```python
from build123d import *

# Parameters (mm, degrees)
SKETCH2_W                            = 83
SKETCH2_H                            = 30
BOSS_EXTRUDE1_DEPTH                  = 120
CUT_EXTRUDE1_DEPTH                   = 28
CUT_EXTRUDE4_REACH                   = 122
SKETCH10_R                           = 3
SKETCH10_R_2                         = 1.6
BOSS_EXTRUDE2_DEPTH                  = 5
SKETCH13_R                           = 5
BOSS_EXTRUDE_CC3D_SUPPORT_DEPTH      = 2
SKETCH10_3_R                         = 1.6
CUT_EXTRUDE_CC3D_ROUND_DEPTH         = 10
CUT_EXTRUDE_CC3D_ROUND_DEPTH_BACK    = 5
SKETCH14_R                           = 1.6
CUT_EXTRUDE_BOTTOM_HEX_CORNERS_DEPTH = 3.5
SKETCH14_5_R                         = 1.6
CUT_EXTRUDE_BOTTOM_HEX_CC3D_DEPTH    = 2.5
SKETCH14_4_R                         = 1.6
CUT_EXTRUDE_BOTTOM_ROUND_DEPTH       = 31
CUT_EXTRUDE12_DEPTH                  = 25
CUT_HOLES_RIGHT_REACH                = 85
SKETCH8_R                            = 4
CUT_HOLES_LEFT_START                 = -83
SKETCH8_4_R                          = 4
CUT_HOLES_LEFT_DEPTH                 = 2
FILLET1_4MM_R                        = 4
CUT_EXTRUDE14_REACH                  = 122
SKETCH15_R                           = 3
CUT_EXTRUDE15_START                  = -120
SKETCH15_2_R                         = 3
CUT_EXTRUDE15_DEPTH                  = 2


with BuildPart() as part:
    # Sketch2 → Boss-Extrude1 (new body)
    with BuildSketch(Plane.XY):
        Rectangle(SKETCH2_W, SKETCH2_H)
    extrude(amount=-BOSS_EXTRUDE1_DEPTH)

    # Sketch4 → Cut-Extrude1 (cut)
    with BuildSketch(Plane(origin=(0, 15, 0), x_dir=(1, 0, 0), z_dir=(0, 1, 0))):
        with BuildLine():
            Line((-24.5, 118), (-31, 118))
            ThreePointArc((-31, 118), (-33.48959236, 111.98959236), (-39.5, 109.5))
            Line((-39.5, 109.5), (-39.5, 10.5))
            ThreePointArc((-39.5, 10.5), (-33.48959236, 8.01040764), (-31, 2))
            Line((-31, 2), (-24.5, 2))
            Line((-24.5, 2), (-24.5, 55))
            Line((-24.5, 55), (-22.5, 55))
            Line((-22.5, 55), (-22.5, 2))
            Line((-22.5, 2), (22.5, 2))
            Line((22.5, 2), (22.5, 55))
            Line((22.5, 55), (24.5, 55))
            Line((24.5, 55), (24.5, 2))
            Line((24.5, 2), (31, 2))
            ThreePointArc((31, 2), (33.48959236, 8.01040764), (39.5, 10.5))
            Line((39.5, 10.5), (39.5, 109.5))
            ThreePointArc((39.5, 109.5), (33.48959236, 111.98959236), (31, 118))
            Line((31, 118), (24.5, 118))
            Line((24.5, 118), (24.5, 65))
            Line((24.5, 65), (22.5, 65))
            Line((22.5, 65), (22.5, 118))
            Line((22.5, 118), (-22.5, 118))
            Line((-22.5, 118), (-22.5, 65))
            Line((-22.5, 65), (-24.5, 65))
            Line((-24.5, 65), (-24.5, 118))
        make_face()
    extrude(amount=-CUT_EXTRUDE1_DEPTH, mode=Mode.SUBTRACT)

    # Sketch6 → Cut-Extrude4 (cut, up to next)
    with BuildSketch(Plane.XY, mode=Mode.PRIVATE) as cut_extrude4_sk1:
        with BuildLine():
            Line((-2, 2), (2, 2))
            ThreePointArc((2, 2), (4, 0), (2, -2))
            Line((2, -2), (-2, -2))
            ThreePointArc((-2, -2), (-4, 0), (-2, 2))
        make_face()
    cut_extrude4_tool1 = extrude(cut_extrude4_sk1.sketch, amount=-CUT_EXTRUDE4_REACH, mode=Mode.PRIVATE) & part.part
    add(cut_extrude4_tool1.solids().sort_by_distance((0, 0, 0))[0], mode=Mode.SUBTRACT)

    # Sketch10 → Boss-Extrude2 (add)
    with BuildSketch(Plane(origin=(0, -13, 0), x_dir=(1, 0, 0), z_dir=(0, 1, 0))):
        with Locations((-15.25, 100.25)):
            Circle(SKETCH10_R)
        with Locations((-15.25, 100.25)):
            Circle(SKETCH10_R_2, mode=Mode.SUBTRACT)
        with Locations((15.25, 100.25)):
            Circle(SKETCH10_R)
        with Locations((15.25, 100.25)):
            Circle(SKETCH10_R_2, mode=Mode.SUBTRACT)
        with Locations((15.25, 69.75)):
            Circle(SKETCH10_R)
        with Locations((15.25, 69.75)):
            Circle(SKETCH10_R_2, mode=Mode.SUBTRACT)
        with Locations((-15.25, 69.75)):
            Circle(SKETCH10_R)
        with Locations((-15.25, 69.75)):
            Circle(SKETCH10_R_2, mode=Mode.SUBTRACT)
    extrude(amount=BOSS_EXTRUDE2_DEPTH)

    # Sketch13 → Boss-Extrude-cc3d-support (add)
    with BuildSketch(Plane(origin=(0, -13, 0), x_dir=(1, 0, 0), z_dir=(0, 1, 0))):
        with Locations((-15.25, 100.25)):
            Circle(SKETCH13_R)
        with Locations((15.25, 100.25)):
            Circle(SKETCH13_R)
        with Locations((-15.25, 69.75)):
            Circle(SKETCH13_R)
        with Locations((15.25, 69.75)):
            Circle(SKETCH13_R)
    extrude(amount=BOSS_EXTRUDE_CC3D_SUPPORT_DEPTH)

    # Sketch10_3 → Cut-Extrude-cc3d-round (cut, two sides)
    with BuildSketch(Plane(origin=(0, -13, 0), x_dir=(1, 0, 0), z_dir=(0, 1, 0))) as cut_extrude_cc3d_round_sk:
        with Locations((-15.25, 100.25)):
            Circle(SKETCH10_3_R)
        with Locations((15.25, 100.25)):
            Circle(SKETCH10_3_R)
        with Locations((-15.25, 69.75)):
            Circle(SKETCH10_3_R)
        with Locations((15.25, 69.75)):
            Circle(SKETCH10_3_R)
    extrude(amount=CUT_EXTRUDE_CC3D_ROUND_DEPTH, mode=Mode.SUBTRACT)
    extrude(cut_extrude_cc3d_round_sk.sketch, amount=-CUT_EXTRUDE_CC3D_ROUND_DEPTH_BACK, mode=Mode.SUBTRACT)

    # Sketch14 → Cut-Extrude-bottom-hex-corners (cut)
    with BuildSketch(Plane.XZ.offset(15)):
        Polygon((-39.5, -113.063655198), (-39.5, -116.354551733), (-36.65, -118), (-33.8, -116.354551733), (-33.8, -113.063655198), (-36.65, -111.418206931), align=None)
        with Locations((-36.65, -114.709103466)):
            Circle(SKETCH14_R, mode=Mode.SUBTRACT)
        Polygon((33.8, -113.063655198), (33.8, -116.354551733), (36.65, -118), (39.5, -116.354551733), (39.5, -113.063655198), (36.65, -111.418206931), align=None)
        with Locations((36.65, -114.709103466)):
            Circle(SKETCH14_R, mode=Mode.SUBTRACT)
        Polygon((33.8, -3.645448267), (33.8, -6.936344802), (36.65, -8.581793069), (39.5, -6.936344802), (39.5, -3.645448267), (36.65, -2), align=None)
        with Locations((36.65, -5.290896534)):
            Circle(SKETCH14_R, mode=Mode.SUBTRACT)
        Polygon((-39.5, -3.645448267), (-39.5, -6.936344802), (-36.65, -8.581793069), (-33.8, -6.936344802), (-33.8, -3.645448267), (-36.65, -2), align=None)
        with Locations((-36.65, -5.290896534)):
            Circle(SKETCH14_R, mode=Mode.SUBTRACT)
    extrude(amount=-CUT_EXTRUDE_BOTTOM_HEX_CORNERS_DEPTH, mode=Mode.SUBTRACT)

    # Sketch14_5 → Cut-Extrude-bottom-hex-cc3d (cut)
    with BuildSketch(Plane.XZ.offset(15)):
        Polygon((-18.1, -98.604551733), (-18.1, -101.895448267), (-15.25, -103.540896534), (-12.4, -101.895448267), (-12.4, -98.604551733), (-15.25, -96.959103466), align=None)
        with Locations((-15.25, -100.25)):
            Circle(SKETCH14_5_R, mode=Mode.SUBTRACT)
        Polygon((-18.1, -68.104551733), (-18.1, -71.395448267), (-15.25, -73.040896534), (-12.4, -71.395448267), (-12.4, -68.104551733), (-15.25, -66.459103466), align=None)
        with Locations((-15.25, -69.75)):
            Circle(SKETCH14_5_R, mode=Mode.SUBTRACT)
        Polygon((12.4, -68.104551733), (12.4, -71.395448267), (15.25, -73.040896534), (18.1, -71.395448267), (18.1, -68.104551733), (15.25, -66.459103466), align=None)
        with Locations((15.25, -69.75)):
            Circle(SKETCH14_5_R, mode=Mode.SUBTRACT)
        Polygon((12.4, -98.604551733), (12.4, -101.895448267), (15.25, -103.540896534), (18.1, -101.895448267), (18.1, -98.604551733), (15.25, -96.959103466), align=None)
        with Locations((15.25, -100.25)):
            Circle(SKETCH14_5_R, mode=Mode.SUBTRACT)
    extrude(amount=-CUT_EXTRUDE_BOTTOM_HEX_CC3D_DEPTH, mode=Mode.SUBTRACT)

    # Sketch14_4 → Cut-Extrude-bottom-round (cut, through all)
    with BuildSketch(Plane.XZ.offset(15)):
        with Locations((-36.65, -5.290896534)):
            Circle(SKETCH14_4_R)
        with Locations((36.65, -5.290896534)):
            Circle(SKETCH14_4_R)
        with Locations((36.65, -114.709103466)):
            Circle(SKETCH14_4_R)
        with Locations((-36.65, -114.709103466)):
            Circle(SKETCH14_4_R)
    extrude(amount=-CUT_EXTRUDE_BOTTOM_ROUND_DEPTH, mode=Mode.SUBTRACT)

    # Sketch4_5 → Cut-Extrude12 (cut)
    with BuildSketch(Plane(origin=(0, 15, 0), x_dir=(1, 0, 0), z_dir=(0, 1, 0))):
        with BuildLine():
            Line((-31, 118), (-39.5, 118))
            Line((-39.5, 118), (-39.5, 109.5))
            ThreePointArc((-39.5, 109.5), (-33.48959236, 111.98959236), (-31, 118))
        make_face()
        with BuildLine():
            Line((39.5, 118), (31, 118))
            ThreePointArc((31, 118), (33.48959236, 111.98959236), (39.5, 109.5))
            Line((39.5, 109.5), (39.5, 118))
        make_face()
        with BuildLine():
            Line((39.5, 2), (39.5, 10.5))
            ThreePointArc((39.5, 10.5), (33.48959236, 8.01040764), (31, 2))
            Line((31, 2), (39.5, 2))
        make_face()
        with BuildLine():
            ThreePointArc((-31, 2), (-33.48959236, 8.01040764), (-39.5, 10.5))
            Line((-39.5, 10.5), (-39.5, 2))
            Line((-39.5, 2), (-31, 2))
        make_face()
    extrude(amount=-CUT_EXTRUDE12_DEPTH, mode=Mode.SUBTRACT)

    # Sketch8 → Cut-Holes-Right (cut, up to next)
    with BuildSketch(Plane(origin=(41.5, 0, 0), x_dir=(0, 0, -1), z_dir=(1, 0, 0)), mode=Mode.PRIVATE) as cut_holes_right_sk1:
        with Locations((30, 0)):
            Circle(SKETCH8_R)
    cut_holes_right_tool1 = extrude(cut_holes_right_sk1.sketch, amount=-CUT_HOLES_RIGHT_REACH, mode=Mode.PRIVATE) & part.part
    add(cut_holes_right_tool1.solids().sort_by_distance((41.5, 0, -30))[0], mode=Mode.SUBTRACT)
    # Sketch8 → Cut-Holes-Right (cut, up to next)
    with BuildSketch(Plane(origin=(41.5, 0, 0), x_dir=(0, 0, -1), z_dir=(1, 0, 0)), mode=Mode.PRIVATE) as cut_holes_right_sk2:
        with Locations((90, 0)):
            Circle(SKETCH8_R)
    cut_holes_right_tool2 = extrude(cut_holes_right_sk2.sketch, amount=-CUT_HOLES_RIGHT_REACH, mode=Mode.PRIVATE) & part.part
    add(cut_holes_right_tool2.solids().sort_by_distance((41.5, 0, -90))[0], mode=Mode.SUBTRACT)

    # Sketch8_4 → Cut-Holes-Left (cut)
    with BuildSketch(Plane(origin=(41.5, 0, 0), x_dir=(0, 0, -1), z_dir=(1, 0, 0)).offset(CUT_HOLES_LEFT_START)):
        with Locations((30, 0)):
            Circle(SKETCH8_4_R)
        with Locations((90, 0)):
            Circle(SKETCH8_4_R)
    extrude(amount=CUT_HOLES_LEFT_DEPTH, mode=Mode.SUBTRACT)

    # Fillet1_4mm
    fillet1_4mm_edges = [part.edges().sort_by_distance(p)[0] for p in [
        (41.5, 0, -120),
        (-39.5, 2.5, -118),
        (39.5, 2.5, -118),
        (39.5, 2.5, -2),
        (-41.5, 0, -120),
        (-39.5, 2.5, -2),
        (41.5, 0, 0),
        (-41.5, 0, 0),
    ]]
    fillet(fillet1_4mm_edges, radius=FILLET1_4MM_R)

    # Sketch15 → Cut-Extrude14 (cut, up to next)
    with BuildSketch(Plane.XY, mode=Mode.PRIVATE) as cut_extrude14_sk1:
        with Locations((-32.5, 0)):
            Circle(SKETCH15_R)
    cut_extrude14_tool1 = extrude(cut_extrude14_sk1.sketch, amount=-CUT_EXTRUDE14_REACH, mode=Mode.PRIVATE) & part.part
    add(cut_extrude14_tool1.solids().sort_by_distance((-32.5, 0, 0))[0], mode=Mode.SUBTRACT)
    # Sketch15 → Cut-Extrude14 (cut, up to next)
    with BuildSketch(Plane.XY, mode=Mode.PRIVATE) as cut_extrude14_sk2:
        with Locations((32.5, 0)):
            Circle(SKETCH15_R)
    cut_extrude14_tool2 = extrude(cut_extrude14_sk2.sketch, amount=-CUT_EXTRUDE14_REACH, mode=Mode.PRIVATE) & part.part
    add(cut_extrude14_tool2.solids().sort_by_distance((32.5, 0, 0))[0], mode=Mode.SUBTRACT)

    # Sketch15_2 → Cut-Extrude15 (cut)
    with BuildSketch(Plane.XY.offset(CUT_EXTRUDE15_START)):
        with Locations((-32.5, 0)):
            Circle(SKETCH15_2_R)
        with Locations((32.5, 0)):
            Circle(SKETCH15_2_R)
    extrude(amount=CUT_EXTRUDE15_DEPTH, mode=Mode.SUBTRACT)


solid = part.part
```
Build history of the part. All positions in model axes, mm. A direction names the side the tool comes from. Round coordinates to 2 decimals unless told otherwise and drop trailing zeros. Loops run counter-clockwise (first coordinate to the right, second up) from the corner with the lowest first, then second, coordinate; pieces in that order, holes last.
Item 1: Saw through at A-A (z = -30). List the corners of the cut face in (x, y), then the cut area to 3 significant figures.
Item 2: Which spindle directions (+Z, -Z, +X, -X, +Y, -Y) get a long thin tool onto all of the face, cutting with end or side? Do faces 1 (the face through (-41, 0, -86)), 2 (the face through (16.69, -13.77, -67.29)), 3 (the face through (-29, 1, -118)). Say none if no direction does.
Item 3: Pin check, flat tips, straight feed: P1, Ø2.5, axis at x = -36.65, z = -5.29, coming from the +Y side; P2, Ø8, axis at x = 0, z = -27, coming from the +Y side; P3, Ø3, axis at x = 15, z = -102.5, coming from the +Y side; P4, Ø4, axis at x = -15.25, z = -69.75, coming from the -Y side. Stop position of each tip, or through.
Item 4: Two-plate mould, pull along Z, no slides. Class faces 4 (the face through (-29, 1, -2)), 5 (the face through (40.297, 0.21, -118.859)), 6 (the face through (29.5, 0.1, -1)): released by +Z, released by -Z, zero draft, split by the parting line, or undercut.
Item 5: Saw through at C-C (x = 6). List the corners of the cut face in (y, z), then the cut area to 3 significant figures.
Item 6: Saw through at D-D (z = -63.5). List the corners of the cut face in (x, y), then the cut area to 3 significant figures.
Item 7: Drill centre lines: line 1 along Z through (x, y) = (-15.25, -11.4); line 2 along X through (y, z) = (-1, -72.5); line 3 along Z through (x, y) = (21.5, -3.5). Where is each one in solid material? Low to high.
Worked answers:
1. outline: (-41.5, -15) - (41.5, -15) - (41.5, -4) - (39.5, -4) - (39.5, -13) - (24.5, -13) - (24.5, 15) - (22.5, 15) - (22.5, -13) - (-22.5, -13) - (-22.5, 15) - (-24.5, 15) - (-24.5, -13) - (-39.5, -13) - (-39.5, -4) - (-41.5, -4) - close; (-41.5, 4) - (-39.5, 4) - (-39.5, 15) - (-41.5, 15) - close; (39.5, 4) - (41.5, 4) - (41.5, 15) - (39.5, 15) - close
1. area: 358 mm2
2. face 1: -X
2. face 2: -Y
2. face 3: +Y
3. P1: passes through
3. P2: stops at y = -13
3. P3: stops at y = -8
3. P4: stops at y = -12.5
4. face 4: undercut
4. face 5: released by -Z
4. face 6: zero draft
5. outline: (-15, -120) - (15, -120) - (15, -118) - (-13, -118) - (-13, -2) - (15, -2) - (15, 0) - (-15, 0) - close
5. area: 352 mm2
6. outline: (-41.5, -15) - (41.5, -15) - (41.5, 15) - (39.5, 15) - (39.5, -13) - (-39.5, -13) - (-39.5, 15) - (-41.5, 15) - close
6. area: 278 mm2
7. line 1: z = -120 to -118, -105.25 to -101.85, -98.65 to -95.25, -74.75 to -71.35, -68.15 to -64.75, -2 to 0
7. line 2: x = -41.5 to -39.5, -24.5 to -22.5, 22.5 to 24.5, 39.5 to 41.5
7. line 3: z = -120 to -118, -2 to 0
